```python
from build123d import *

# Parameters (mm, degrees)
SKETCH006_R      = 1.25
EXTRUDE008_DEPTH = 2
EXTRUDE005_DEPTH = 20
SKETCH_R         = 20
SKETCH_R_2       = 18
EXTRUDE_DEPTH    = 70


with BuildPart() as extrude008:
    # Sketch006 → Extrude008 (new body)
    with BuildSketch(Plane(origin=(20, 0, 12), x_dir=(0, 1, 0), z_dir=(1, 0, 0))):
        Circle(SKETCH006_R)
        with Locations((-0.013333, 3.999978)):
            Circle(SKETCH006_R)
        with Locations((-0.026665, 7.999956)):
            Circle(SKETCH006_R)
        with Locations((-0.039998, 11.999933)):
            Circle(SKETCH006_R)
        with Locations((-0.053331, 15.999911)):
            Circle(SKETCH006_R)
        with Locations((-0.066663, 19.999889)):
            Circle(SKETCH006_R)
        with Locations((-0.079996, 23.999867)):
            Circle(SKETCH006_R)
        with Locations((-0.093328, 27.999844)):
            Circle(SKETCH006_R)
        with Locations((-0.106661, 31.999822)):
            Circle(SKETCH006_R)
        with Locations((-0.119994, 35.9998)):
            Circle(SKETCH006_R)
        with Locations((-0.133326, 39.999778)):
            Circle(SKETCH006_R)
        with Locations((-0.146659, 43.999756)):
            Circle(SKETCH006_R)
        with Locations((-0.159992, 47.999733)):
            Circle(SKETCH006_R)
        with Locations((-0.173324, 51.999711)):
            Circle(SKETCH006_R)
    extrude(amount=-EXTRUDE008_DEPTH)


with BuildPart() as extrude005:
    # Sketch004 → Extrude005 (new body, symmetric)
    with BuildSketch(Plane.YZ):
        with BuildLine():
            Line((2, 4), (2, 0))
            Line((2, 0), (-2, 0))
            Line((-2, 0), (-2, 4))
            ThreePointArc((2, 4), (0, 6), (-2, 4))
        make_face()
    extrude(amount=EXTRUDE005_DEPTH, both=True)


with BuildPart() as extrude005_1:
    # Extrude005 placement: moved
    add(extrude005.part.moved(Location((10, 0, 0))))


with BuildPart() as cut001:
    # Sketch → Extrude (new body)
    with BuildSketch(Plane.XY):
        Circle(SKETCH_R)
        Circle(SKETCH_R_2, mode=Mode.SUBTRACT)
    extrude(amount=EXTRUDE_DEPTH)

    # Cut: cut Extrude005
    add(extrude005_1.part, mode=Mode.SUBTRACT)

    # Cut001: cut Extrude008
    add(extrude008.part, mode=Mode.SUBTRACT)


solid = cut001.part
```
The listing builds one solid part. Answer for the finished solid, in the listing's coordinates (mm). A direction names the side the tool comes from. Round coordinates to 2 decimals unless told otherwise and drop trailing zeros. Order: outer loops, then holes, each group sorted by start corner. A loop starts at its lowest first (then second) coordinate and runs counter-clockwise, first axis right, second up. Notation, with made-up numbers: (1.25, 52) - (11.25, 52) arc R19 ccw to (11.25, 80) - close; hole circle Ø4 at (25.25, -32.5). An arc over 180 degrees is marked (long way). Put each result on its own line as item: value. Start each with the question number.
(1) For faces 4 (the cylindrical face through (-2.343, 17.847, 34.51)), 5 (the cylindrical face through (19.01, -0.34, 65.24)), determine the directions among +Z, -Z, +X, -X, +Y, -Y from which every point of the face is accessible in a straight line to the end or side of a thin tool.
(2) Find section B-B (y = 9.5). Give the vertices of the cut face in (x, z), plus the area to 3 significant figures.
(3) Find section A-A (x = 0). Give the vertices of the cut face in (y, z), plus the area to 3 significant figures.
(4) Determine the mould class of faces 1 (the cylindrical face through (19, 0, 6)), 2 (the flat face through (19, -2, 2)), 3 (the cylindrical face through (19.01, -0.23, 33.24)) for opening direction Z: released by +Z, released by -Z, zero draft, split by the parting line, or undercut.
(5) Find section C-C (z = 46). Give the vertices of the cut face in (x, y), plus the area to 3 significant figures.
(6) Given P1, Ø2, axis at y = -0.07, z = 32, coming from the +X side; P2, Ø2, axis at x = 15, z = 16, coming from the -Y side; P3, Ø1, axis at x = -8, z = 62, coming from the +Y side; P4, Ø3, axis at y = -0.17, z = 64, coming from the -X side, each flat-ended and moving along its own axis, determine where each tip first touches the part or whether it passes through.
(7) Straight lines are drawn through the part: probe 1 along X at (y, z) = (11, 41.5); probe 2 along X at (y, z) = (-1, 42); probe 3 along Y at (x, z) = (6, 28). For each, find the intervals that lie inside material, in ascending order. Write a range as from..to.
Reply:
1. face 4: +Z, -Z
1. face 5: +X
2. outline: (-17.6, 0) - (-15.29, 0) - (-15.29, 70) - (-17.6, 70) - close; (15.29, 0) - (17.6, 0) - (17.6, 70) - (15.29, 70) - close
2. area: 324 mm^2
3. outline: (-20, 0) - (-18, 0) - (-18, 70) - (-20, 70) - close; (18, 0) - (20, 0) - (20, 70) - (18, 70) - close
3. area: 280 mm^2
4. face 1: released by -Z
4. face 2: zero draft
4. face 3: undercut
5. outline: circle Ø40 at (0, 0); hole circle Ø36 at (0, 0)
5. area: 239 mm^2
6. P1: x = 18
6. P2: y = -14.28
6. P3: y = 18.54
6. P4: x = -20
7. probe 1: -16.7..-14.25, 14.25..16.7
7. probe 2: -19.97..-17.97, 17.97..19.97
7. probe 3: -19.08..-16.97, 16.97..19.08
